Source: CAD feature listing. Evaluate the final solid. Frame: model axes, mm. Face numbers are marked on the shaded views. Round coordinates to 2 decimals unless told otherwise and drop trailing zeros. Order: outer loops, then holes, each group sorted by start corner. A loop starts at its lowest first (then second) coordinate and runs counter-clockwise, first axis right, second up. Notation, with made-up numbers: (68, 59.25) - (90, 59.25) arc R20 cw to (90, 91.25) - close; hole circle Ø3 at (37.25, 82). An arc over 180 degrees is marked (long way). Put each result on its own line as item: value. Start each with the question number.
1) Contact query for flat-ended pins moving along their axis: P1, Ø1, axis at x = -1, z = 2, coming from the +Y side; P2, Ø1.5, axis at y = 1.5, z = 4.5, coming from the -X side. Output: stop coordinate, or through.
2) Line query: probe 1 along X at (y, z) = (0, 3.9); probe 2 along Z at (x, y) = (2, 1.7); probe 3 along Y at (x, z) = (1.1, 3.15). Output: solid intervals per line, ascending. Write a range as [from, to].
3) Section A-A on y = 0. Output: boundary loops of the cut face in (x, z), then the cut area to 3 significant figures.
4) Section C-C on z = 2.25. Output: boundary loops of the cut face in (x, y), then the cut area to 3 significant figures.
5) Mould query, pull axis Y, two halves, no side actions, for the marked faces 1, 2, 3 and 4. Classes: +Y half, -Y half, draft (parallel to the pull), parting line (faces both ways), or undercut.
Autodesk Inventor part; units mm, degrees
ref_plane "YZ Plane" through (0, 0, 0) normal (1, 0, 0) x (0, 1, 0)
ref_plane "XZ Plane" through (0, 0, 0) normal (0, 1, 0) x (-1, 0, 0)
ref_plane "XY Plane" through (0, 0, 0) normal (0, 0, 1) x (1, 0, 0)
sketch "Skizze3" plane through (0, 0, 0) normal (1, 0, 0) x (0, 1, 0)
  line L0 (0, 0) -> (0, 9.4008)
  line L1 (-1, 0) -> (-1, 1.5)
  line L2 (-1, 1.5) -> (-1.75, 1.5)
  line L3 (-1.75, 1.5) -> (-1.75, 6)
  line L4 (-1.75, 6) -> (-3, 6)
  line L5 (-2.5, 0) -> (0, 0)
  line L6 (-3, 6) -> (-3, 1)
  line L7 (-3, 1) -> (-2.5, 1)
  line L8 (-2.5, 1) -> (-2.5, 0)
  dimension "d4" = 2
  dimension "d5" = 1.5
  dimension "d6" = 3.5
  dimension "d8" = 5
  dimension "d9" = 6
  dimension "d10" = 1
  dimension "d11" = 6
revolve "Umdrehung1" add sketch "Skizze3" angle 360 about axis through (0, 0, 0) along (0, 0, 1)
chamfer "Fase1" distance 0.2 angle 45 4 edges at (0, 1.75, 6) (0, 2.5, 0) (0, 3, 1) (0, 3, 6)
thread "Gewinde2"
properties part number "BT004_huenin20_23" material "Kupfer"
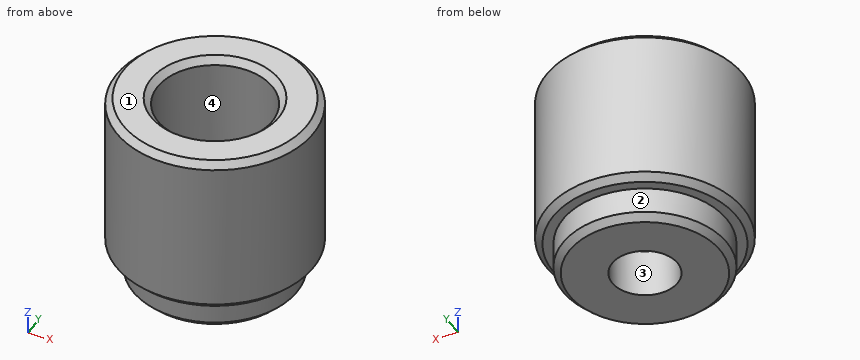
Answer sheet:
1. P1: y = 2.96
1. P2: x = -2.9
2. probe 1: [-3, -1.75], [1.75, 3]
2. probe 2: [1, 6]
2. probe 3: [-2.79, -1.36], [1.36, 2.79]
3. outline: (-3, 1.2) - (-2.8, 1) - (-2.5, 1) - (-2.5, 0.2) - (-2.3, 0) - (-1, 0) - (-1, 1.5) - (-1.75, 1.5) - (-1.75, 5.8) - (-1.95, 6) - (-2.8, 6) - (-3, 5.8) - close; (1, 0) - (2.3, 0) - (2.5, 0.2) - (2.5, 1) - (2.8, 1) - (3, 1.2) - (3, 5.8) - (2.8, 6) - (1.95, 6) - (1.75, 5.8) - (1.75, 1.5) - (1, 1.5) - close
3. area: 16.1 mm^2
4. outline: circle Ø6 at (0, 0); hole circle Ø3.5 at (0, 0)
4. area: 18.7 mm^2
5. face 1: draft
5. face 2: parting line
5. face 3: undercut
5. face 4: undercut
